The listing builds one solid part. Answer for the finished solid, in the listing's coordinates (mm). A direction names the side the tool comes from. Coordinates: 2 decimals unless noted, no trailing zeros. Order: outer loops, then holes, each group sorted by start corner. A loop starts at its lowest first (then second) coordinate and runs counter-clockwise, first axis right, second up. Notation, with made-up numbers: (78.25, 25.5) -> (87.25, 25.5) arc R12 cw to (87.25, 47.5) -> close; hole circle Ø9 at (83, -1). An arc over 180 degrees is marked (long way). Return JSON: item names as keys, results as strings.
from build123d import *

# Parameters (mm, degrees)
SKETCH1_W           = 282.5
SKETCH1_H           = 150.5
BOSS_EXTRUDE2_DEPTH = 105
SKETCH16_W          = 80
SKETCH16_H          = 40
SKETCH16_W_2        = 130
SKETCH16_H_2        = 45.5
CUT_EXTRUDE10_DEPTH = 105
SKETCH17_W          = 20
SKETCH17_H          = 32.5
CUT_EXTRUDE11_DEPTH = 110.5
CUT_EXTRUDE12_DEPTH = 90.5
SKETCH19_W          = 92.5
SKETCH19_H          = 50
CUT_EXTRUDE13_DEPTH = 14
SKETCH20_W          = 92.5
SKETCH20_H          = 50
CUT_EXTRUDE14_DEPTH = 14
SKETCH21_W          = 25
SKETCH21_H          = 50
CUT_EXTRUDE15_DEPTH = 85
SKETCH22_W          = 85
SKETCH22_H          = 85
CUT_EXTRUDE16_DEPTH = 105
CUT_EXTRUDE17_DEPTH = 50
CUT_EXTRUDE18_DEPTH = 120
CUT_EXTRUDE19_DEPTH = 50
SKETCH27_R          = 5
CUT_EXTRUDE20_DEPTH = 120
CUT_EXTRUDE21_DEPTH = 160
FILLET1_R           = 10
FILLET2_R           = 10
CUT_EXTRUDE22_DEPTH = 160
FILLET3_R           = 10
SKETCH30_W          = 20
SKETCH30_H          = 20
CUT_EXTRUDE23_DEPTH = 160


with BuildPart() as part:
    # Sketch1 → Boss-Extrude2 (new body)
    with BuildSketch(Plane.XY):
        with Locations((93.419387358, 47.520353684)):
            Rectangle(SKETCH1_W, SKETCH1_H)
    extrude(amount=BOSS_EXTRUDE2_DEPTH)

    # Sketch16 → Cut-Extrude10 (cut)
    with BuildSketch(Plane.XY.offset(105)):
        with Locations((194.669387358, -7.729646316)):
            Rectangle(SKETCH16_W, SKETCH16_H)
        with Locations((17.169387358, 100.020353684)):
            Rectangle(SKETCH16_W_2, SKETCH16_H_2)
    extrude(amount=-CUT_EXTRUDE10_DEPTH, mode=Mode.SUBTRACT)

    # Sketch17 → Cut-Extrude11 (cut)
    with BuildSketch(Plane(origin=(0, 122.770353684, 0), x_dir=(1, 0, 0), z_dir=(0, 1, 0))):
        with Locations((224.669387358, -16.25)):
            Rectangle(SKETCH17_W, SKETCH17_H)
        with Locations((224.669387358, -88.75)):
            Rectangle(SKETCH17_W, SKETCH17_H)
    extrude(amount=-CUT_EXTRUDE11_DEPTH, mode=Mode.SUBTRACT)

    # Sketch18 → Cut-Extrude12 (cut)
    with BuildSketch(Plane(origin=(0, 122.770353684, 0), x_dir=(1, 0, 0), z_dir=(0, 1, 0))):
        Polygon((214.669387358, -32.5), (194.669387358, -32.5), (194.669387358, -50), (82.169387358, -50), (82.169387358, 0), (214.669387358, 0), align=None)
        Polygon((214.669387358, -72.5), (194.669387358, -72.5), (194.669387358, -55), (82.169387358, -55), (82.169387358, -105), (214.669387358, -105), align=None)
    extrude(amount=-CUT_EXTRUDE12_DEPTH, mode=Mode.SUBTRACT)

    # Sketch19 → Cut-Extrude13 (cut)
    with BuildSketch(Plane(origin=(0, 32.270353684, 0), x_dir=(1, 0, 0), z_dir=(0, 1, 0))):
        with Locations((128.419387358, -80)):
            Rectangle(SKETCH19_W, SKETCH19_H)
    extrude(amount=-CUT_EXTRUDE13_DEPTH, mode=Mode.SUBTRACT)

    # Sketch20 → Cut-Extrude14 (cut)
    with BuildSketch(Plane(origin=(0, 32.270353684, 0), x_dir=(1, 0, 0), z_dir=(0, 1, 0))):
        with Locations((128.419387358, -25)):
            Rectangle(SKETCH20_W, SKETCH20_H)
    extrude(amount=-CUT_EXTRUDE14_DEPTH, mode=Mode.SUBTRACT)

    # Sketch21 → Cut-Extrude15 (cut)
    with BuildSketch(Plane(origin=(0, 77.270353684, 0), x_dir=(1, 0, 0), z_dir=(0, 1, 0))):
        with Locations((69.669387358, -25)):
            Rectangle(SKETCH21_W, SKETCH21_H)
        with Locations((69.669387358, -80)):
            Rectangle(SKETCH21_W, SKETCH21_H)
    extrude(amount=-CUT_EXTRUDE15_DEPTH, mode=Mode.SUBTRACT)

    # Sketch22 → Cut-Extrude16 (cut)
    with BuildSketch(Plane(origin=(0, 77.270353684, 0), x_dir=(1, 0, 0), z_dir=(0, 1, 0))):
        with Locations((4.669387358, -52.5)):
            Rectangle(SKETCH22_W, SKETCH22_H)
    extrude(amount=-CUT_EXTRUDE16_DEPTH, mode=Mode.SUBTRACT)

    # Sketch24 → Cut-Extrude17 (cut)
    with BuildSketch(Plane.XY.offset(105)):
        Polygon((151.871541409, 18.270353684), (118.307556162, -21.729646316), (82.169387358, -21.729646316), (82.169387358, -7.729646316), (82.169387358, 18.270353684), align=None)
    extrude(amount=-CUT_EXTRUDE17_DEPTH, mode=Mode.SUBTRACT)

    # Sketch25 → Cut-Extrude18 (cut)
    with BuildSketch(Plane.XY.offset(105)):
        Polygon((154.669387358, -27.729646316), (154.669387358, 12.270353684), (121.105402111, -27.729646316), align=None)
    extrude(amount=-CUT_EXTRUDE18_DEPTH, mode=Mode.SUBTRACT)

    # Sketch26 → Cut-Extrude19 (cut)
    with BuildSketch(Plane(origin=(0, 0, 0), x_dir=(-1, 0, 0), z_dir=(0, 0, -1))):
        Polygon((-82.169387358, -7.729646316), (-82.169387358, -21.729646316), (-118.307556162, -21.729646316), (-151.871541409, 18.270353684), (-82.169387358, 18.270353684), align=None)
    extrude(amount=-CUT_EXTRUDE19_DEPTH, mode=Mode.SUBTRACT)

    # Sketch27 → Cut-Extrude20 (cut)
    with BuildSketch(Plane(origin=(0, 0, 0), x_dir=(-1, 0, 0), z_dir=(0, 0, -1))):
        with Locations((-184.669387358, 22.270353684)):
            Circle(SKETCH27_R)
        with Locations((-72.169387358, -17.729646316)):
            Circle(SKETCH27_R)
    extrude(amount=-CUT_EXTRUDE20_DEPTH, mode=Mode.SUBTRACT)

    # Sketch28 → Cut-Extrude21 (cut)
    with BuildSketch(Plane.XZ.offset(27.729646316)):
        Polygon((10.669387358, 105), (214.669387358, 105), (214.669387358, 72.5), align=None)
        Polygon((214.669387358, 32.5), (10.669387358, 0), (214.669387358, 0), align=None)
    extrude(amount=-CUT_EXTRUDE21_DEPTH, mode=Mode.SUBTRACT)

    # Fillet1
    fillet1_edges = [part.edges().sort_by_distance(p)[0] for p in [
        (174.669387358, 32.270353684, 38.06372549),
        (82.169387358, -7.729646316, 30.695465686),
        (82.169387358, -7.729646316, 74.304534314),
        (174.669387358, 32.270353684, 66.93627451),
    ]]
    fillet(fillet1_edges, radius=FILLET1_R)

    # Fillet2
    fillet2_edges = [part.edges().sort_by_distance(p)[0] for p in [
        (151.871541409, 18.270353684, 68.752279395),
        (118.307556162, -21.729646316, 71.425881161),
        (151.871541409, 18.270353684, 36.247720605),
        (118.307556162, -21.729646316, 33.574118839),
        (154.669387358, 12.270353684, 52.5),
        (121.105402111, -27.729646316, 52.5),
    ]]
    fillet(fillet2_edges, radius=FILLET2_R)

    # Sketch29 → Cut-Extrude22 (cut)
    with BuildSketch(Plane.XY.offset(55)):
        Polygon((82.169387358, 77.270353684), (140.676980695, 77.270353684), (178.856013913, 122.770353684), (82.169387358, 122.770353684), align=None)
    extrude(amount=-CUT_EXTRUDE22_DEPTH, mode=Mode.SUBTRACT)

    # Fillet3
    fillet3_edges = [part.edges().sort_by_distance(p)[0] for p in [
        (178.856013913, 122.770353684, 52.5),
        (140.676980695, 77.270353684, 52.5),
    ]]
    fillet(fillet3_edges, radius=FILLET3_R)

    # Sketch30 → Cut-Extrude23 (cut)
    with BuildSketch(Plane(origin=(0, 122.770353684, 0), x_dir=(1, 0, 0), z_dir=(0, 1, 0))):
        with Locations((214.669387358, -52.5)):
            Rectangle(SKETCH30_W, SKETCH30_H)
    extrude(amount=-CUT_EXTRUDE23_DEPTH, mode=Mode.SUBTRACT)


solid = part.part
1. Consider line 1 (X direction, y = 28, z = 51); line 2 (X direction, y = 64.5, z = 34.5); line 3 (X direction, y = 11.5, z = 94). Determine where each line is inside the solid, lowest interval first. Write a range as from..to.
Answer block:
{"line 1": "x = -47.83..-37.83, 47.17..204.67, 224.67..234.67", "line 2": "x = -47.83..-37.83, 47.17..57.17, 194.67..234.67", "line 3": "x = -47.83..-37.83, 47.17..57.17"}
2. Each of these flat-tipped pins is pushed along its axis until it touches: pin 1 Ø10 at (x, y) = (211, 82) entering from -Z; pin 2 Ø16 at (y, z) = (90, 55) entering from -X; pin 3 Ø1 at (x, z) = (163.5, 29.5) entering from -Y. Where does it stop, or does it pass through?
Answer block:
{"pin 1": "stops at z = 32.5", "pin 2": "stops at x = 144.65", "pin 3": "stops at y = 12.27"}
3. The part is cut by section B-B on y = 63.5. Give the vertices of the cut face in (x, z).
Answer block:
{"outline": "(-47.83, 0) -> (10.67, 0) -> (57.17, 7.41) -> (57.17, 50) -> (194.67, 50) -> (194.67, 32.5) -> (234.67, 32.5) -> (234.67, 72.5) -> (194.67, 72.5) -> (194.67, 55) -> (57.17, 55) -> (57.17, 97.59) -> (10.67, 105) -> (-47.83, 105) -> close; hole (-37.83, 10) -> (47.17, 10) -> (47.17, 95) -> (-37.83, 95) -> close; hole (204.67, 42.5) -> (224.67, 42.5) -> (224.67, 62.5) -> (204.67, 62.5) -> close"}
4. The part is cut by section A-A on z = 59. Give the number of separate pieces and of enclosed holes in the cut face, and give its area (3 significant figures).
Answer block:
{"separate pieces": "3", "enclosed holes": "2", "area": "5,680 mm2"}
5. Determine the mould class of faces 1 (the face through (134.897, -1.96, 33.586)), 2 (the face through (51, -27.73, 52)), 3 (the face through (52.701, 20.636, 6.696)), 4 (the face through (69.5, -13.5, 51.9)) for opening direction Y: pulls with the +Y half, pulls with the -Y half, needs draft (parallel to the pull), parting line crosses it, or undercut.
Answer block:
{"face 1": "pulls with the +Y half", "face 2": "pulls with the -Y half", "face 3": "needs draft", "face 4": "undercut"}
6. The part is cut by section D-D on y = 108.5. Give the vertices of the cut face in (x, z).
Answer block:
{"outline": "(166.88, 50) -> (194.67, 50) -> (194.67, 32.5) -> (234.67, 32.5) -> (234.67, 72.5) -> (194.67, 72.5) -> (194.67, 55) -> (166.88, 55) -> close; hole (204.67, 42.5) -> (224.67, 42.5) -> (224.67, 62.5) -> (204.67, 62.5) -> close"}
7. For faces 5 (the face through (215, 68, 62.5)), 6 (the face through (214, 68, 72.5)), 7 (the face through (152.253, 17.307, 68.795)), determine the directions among +Z, -Z, +X, -X, +Y, -Y from which every point of the face is accessible in a straight line to the end or side of a thin tool.
Answer block:
{"face 5": "+Y, -Y", "face 6": "+Z, +X, +Y", "face 7": "+Z, +Y"}
8. The part is cut by section C-C on x = 37. Give the vertices of the cut face in (y, z), and give its area (3 significant figures).
Answer block:
{"outline": "(-27.73, 4.19) -> (77.27, 4.19) -> (77.27, 10) -> (-27.73, 10) -> close; (-27.73, 95) -> (77.27, 95) -> (77.27, 100.81) -> (-27.73, 100.81) -> close", "area": "1,220 mm2"}
